Can you work these out from the model? Positions are in its coordinate system, mm. A direction names the side the tool comes from. Coordinates: 2 decimals unless noted, no trailing zeros. Order: outer loops, then holes, each group sorted by start corner. A loop starts at its lowest first (then second) coordinate and runs counter-clockwise, first axis right, second up. Notation, with made-up numbers: (66, 89.25) - (101, 89.25) arc R26 ccw to (101, 106.25) - close; hole circle Ø11 at (60, 87). An arc over 180 degrees is marked (long way). Use a Markdown table: item, result. Add a question column.
(1) For pin 1 Ø10 at (x, z) = (0, 0) entering from +Y; pin 2 Ø11 at (y, z) = (0, 0) entering from -X; pin 3 Ø3 at (x, y) = (0, -7.5) entering from -Z; pin 4 Ø4 at (x, y) = (12, 1.5) entering from +Z, each with a flat end and sliding along its axis, tell me the tip position at first contact or that it passes through.
(2) We'd pull the mould along X, two halves only. Please class faces 4 (the flat face through (0, 12.5, 0)), 5 (the cylindrical face through (18.475, 0.35, 7.66)), 6 (the flat face through (4, 25, -5)): pulls with the +X half, pulls with the -X half, needs draft (parallel to the pull), parting line crosses it, or undercut.
(3) I want a section at C-C (z = 4.5). List the corners of the cut face in (x, y) for me, and give its area (3 significant figures).
(4) If I drill on L1, parallel to Y at x = 4.75, z = 0; L2, parallel to X at y = -16.75, z = 0; L3, parallel to Y at x = -15.5, z = 0, over which ranges is the centre line in solid material (lowest first)? Write a range as [from, to].
(5) I want a section at B-B (x = 8). List the corners of the cut face in (y, z) for me, and give its area (3 significant figures).
(6) I want a section at A-A (z = 0). List the corners of the cut face in (x, y) for me.
(7) I want a section at D-D (y = 0). List the corners of the cut face in (x, z) for me.
(8) On a 3-axis mill with a long thin cutter (end or side, diameter ignored), from which of +Z, -Z, +X, -X, +Y, -Y can I reach the whole of each face in a straight line? I mean faces 1 (the flat face through (4, -25, -5)), 2 (the cylindrical face through (5.96, 18.84, -1.88)), 3 (the cylindrical face through (5.96, -18.84, -1.88)). Say none if no direction works.
```python
from build123d import *

# Parameters (mm, degrees)
SKETCH2_R                = 20
BOSS_EXTRUDE1_DEPTH      = 25
BOSS_EXTRUDE1_DEPTH_BACK = 25
SKETCH3_R                = 6.25
CUT_EXTRUDE1_DEPTH       = 40
CUT_EXTRUDE1_DEPTH_BACK  = 40
SKETCH4_R                = 6.25
CUT_EXTRUDE2_DEPTH       = 12.5


with BuildPart() as part:
    # Sketch2 → Boss-Extrude1 (new body, two sides)
    with BuildSketch(Plane(origin=(0, 0, 0), x_dir=(1, 0, 0), z_dir=(0, 1, 0))) as boss_extrude1_sk:
        Circle(SKETCH2_R)
    extrude(amount=BOSS_EXTRUDE1_DEPTH)
    extrude(boss_extrude1_sk.sketch, amount=-BOSS_EXTRUDE1_DEPTH_BACK)

    # Sketch3 → Cut-Extrude1 (cut, two sides)
    with BuildSketch(Plane(origin=(0, 0, 0), x_dir=(0, 0, -1), z_dir=(1, 0, 0))) as cut_extrude1_sk:
        Circle(SKETCH3_R)
    extrude(amount=CUT_EXTRUDE1_DEPTH, mode=Mode.SUBTRACT)
    extrude(cut_extrude1_sk.sketch, amount=-CUT_EXTRUDE1_DEPTH_BACK, mode=Mode.SUBTRACT)

    # Sketch4 → Cut-Extrude2 (cut)
    with BuildSketch(Plane(origin=(0, 25, 0), x_dir=(1, 0, 0), z_dir=(0, 1, 0))):
        Circle(SKETCH4_R)
    cut_extrude2 = extrude(amount=-CUT_EXTRUDE2_DEPTH, mode=Mode.SUBTRACT)

    # Mirror1: Cut-Extrude2 across plane
    add(cut_extrude2.mirror(Plane.ZX), mode=Mode.SUBTRACT)


solid = part.part
```
Answers follow:
| question | item | result |
|---|---|---|
| 1 | pin 1 | stops at y = 12.5 |
| 1 | pin 2 | passes through |
| 1 | pin 3 | stops at z = -20 |
| 1 | pin 4 | stops at z = 17.32 |
| 2 | face 4 | undercut |
| 2 | face 5 | parting line crosses it |
| 2 | face 6 | needs draft |
| 3 | outline | (-19.49, -25) - (-4.34, -25) - (-4.34, -12.5) - (4.34, -12.5) - (4.34, -25) - (19.49, -25) - (19.49, -4.34) - (-19.49, -4.34) - close; (-19.49, 4.34) - (19.49, 4.34) - (19.49, 25) - (4.34, 25) - (4.34, 12.5) - (-4.34, 12.5) - (-4.34, 25) - (-19.49, 25) - close |
| 3 | area | 1,390 mm² |
| 4 | L1 | y = [-12.5, -6.25], [6.25, 12.5] |
| 4 | L2 | x = [-20, -6.25], [6.25, 20] |
| 4 | L3 | y = [-25, -6.25], [6.25, 25] |
| 5 | outline | (-25, -18.33) - (25, -18.33) - (25, 18.33) - (-25, 18.33) - close; hole circle Ø12.5 at (0, 0) |
| 5 | area | 1,710 mm² |
| 6 | outline | (-20, -25) - (-6.25, -25) - (-6.25, -12.5) - (6.25, -12.5) - (6.25, -25) - (20, -25) - (20, -6.25) - (-20, -6.25) - close; (-20, 6.25) - (20, 6.25) - (20, 25) - (6.25, 25) - (6.25, 12.5) - (-6.25, 12.5) - (-6.25, 25) - (-20, 25) - close |
| 7 | outline | (-19, -6.25) arc R20 ccw to (19, -6.25) - close; (-19, 6.25) - (19, 6.25) arc R20 ccw to start |
| 8 | face 1 | +Z, -Z, +X, -X, -Y |
| 8 | face 2 | +Y |
| 8 | face 3 | -Y |
